```python
from build123d import *

# Parameters (mm, degrees)
F0_R          = 11.1125
F1_DEPTH      = 44.45
F2_R          = 6.35
F3_DEPTH      = 88.9
F4_R          = 1.778
F5_DEPTH      = 11.1135
F5_DEPTH_BACK = 11.1135


with BuildPart() as f1:
    # F0 (on Top) → F1 (new body, symmetric)
    with BuildSketch(Plane.XY):
        Circle(F0_R)
    extrude(amount=F1_DEPTH, both=True)

    # F2 (on face) → F3 (cut, through all)
    with BuildSketch(Plane.XY.offset(44.45)):
        Circle(F2_R)
    extrude(amount=-F3_DEPTH, mode=Mode.SUBTRACT)

    # F4 (on Right) → F5 (cut, two sides)
    with BuildSketch(Plane.YZ) as f5_sk:
        with Locations((0, -13.97)):
            Circle(F4_R)
        with Locations((0, 13.97)):
            Circle(F4_R)
    extrude(amount=F5_DEPTH, mode=Mode.SUBTRACT)
    extrude(f5_sk.sketch, amount=-F5_DEPTH_BACK, mode=Mode.SUBTRACT)


solid = f1.part
```
Part model, mm, in its own coordinate system. Round coordinates to 2 decimals unless told otherwise and drop trailing zeros. Write each loop counter-clockwise with the first axis right and the second up, starting at its lowest first coordinate (ties: lowest second). Pieces come first, ordered by that corner, then holes. Notation, with made-up numbers: M 28.5,3 L 76.5,3 A37 cw 76.5,42 Z; hole C 25,-11.75 d1. An arc over 180 degrees is marked long. Answer as CSV lines item,"result". Start each with the question number.
1) Drop flat-ended pins along their axis: pin 1 (2 mm diameter, centred on y = -5.5, z = 21, fed in from -X); pin 2 (4 mm diameter, centred on x = 2.5, z = 13.5, fed in from -Y). Give the stop position or say it passes through.
2) Drill centre lines: L1, parallel to Z at x = 7.5, y = 0; L2, parallel to X at y = 0.5, z = 7; L3, parallel to Z at x = -7, y = 1.5. Where is each one in solid material? Low to high.
3) Band-saw the part on A-A (x = 0). List the corners of the cut face in (y, z), then the cut area to 3 significant figures.
4) Mould opens along Y. For faces 1 (the face through (10.6, 3.34, 0.62)), 2 (the face through (5, -5, 44.45)), 3 (the face through (-8.57, -0.385, 12.234)) say: +Y half, -Y half, draft (parallel to the pull), parting line (faces both ways), or undercut.
5) Band-saw the part on D-D (x = -8.75). List the corners of the cut face in (y, z).
6) Band-saw the part on B-B (y = 0). List the corners of the cut face in (x, z).
Worked out:
1,pin 1,"x = -10.16"
1,pin 2,"y = -11.1"
2,L1,"-44.45 to -15.75, -12.19 to 12.19, 15.75 to 44.45"
2,L2,"-11.1 to -6.33, 6.33 to 11.1"
2,L3,"-44.45 to -14.92, -13.02 to 13.02, 14.92 to 44.45"
3,outline,"M -11.11,-44.45 L -6.35,-44.45 L -6.35,44.45 L -11.11,44.45 Z; M 6.35,-44.45 L 11.11,-44.45 L 11.11,44.45 L 6.35,44.45 Z"
3,area,"847 mm²"
4,face 1,"parting line"
4,face 2,"draft"
4,face 3,"undercut"
5,outline,"M -6.85,-44.45 L 6.85,-44.45 L 6.85,44.45 L -6.85,44.45 Z; hole C 0,-13.97 d3.56; hole C 0,13.97 d3.56"
6,outline,"M -11.11,-44.45 L -6.35,-44.45 L -6.35,-15.75 L -11.11,-15.75 Z; M -11.11,-12.19 L -6.35,-12.19 L -6.35,12.19 L -11.11,12.19 Z; M -11.11,15.75 L -6.35,15.75 L -6.35,44.45 L -11.11,44.45 Z; M 6.35,-44.45 L 11.11,-44.45 L 11.11,-15.75 L 6.35,-15.75 Z; M 6.35,-12.19 L 11.11,-12.19 L 11.11,12.19 L 6.35,12.19 Z; M 6.35,15.75 L 11.11,15.75 L 11.11,44.45 L 6.35,44.45 Z"
